Model file for the job. Use its own axes, mm. A direction names the side the tool comes from. Round coordinates to 2 decimals unless told otherwise and drop trailing zeros. Write each loop counter-clockwise with the first axis right and the second up, starting at its lowest first coordinate (ties: lowest second). Pieces come first, ordered by that corner, then holes. Notation, with made-up numbers: (-30, 55.5) - (14, 55.5) arc R21 ccw to (14, 88.5) - close; hole circle Ø8 at (71, -6.75). An arc over 180 degrees is marked (long way). Answer as a JSON object with one key per item and string values. Group by question number.
from build123d import *

# Parameters (mm, degrees)
SKETCH1_R      = 4.0005
SKETCH1_R_2    = 1.1938
EXTRUDE1_DEPTH = 1.524


with BuildPart() as part:
    # Sketch1 → Extrude1 (new body)
    with BuildSketch(Plane(origin=(0, 0, 0), x_dir=(1, 0, 0), z_dir=(0, 1, 0))):
        with BuildLine():
            Line((0, 3.175), (0, 9.525))
            Line((0, 9.525), (7.9248, 9.525))
            Line((7.9248, 9.525), (7.9248, 3.5814))
            Line((7.9248, 3.5814), (11.557, 3.5814))
            Line((11.557, 3.5814), (11.557, 9.525))
            Line((11.557, 9.525), (20.6756, 9.525))
            Line((20.6756, 9.525), (20.6756, 50.8))
            Line((20.6756, 50.8), (11.557, 50.8))
            Line((11.557, 50.8), (11.557, 56.7436))
            Line((11.557, 56.7436), (7.9248, 56.7436))
            Line((7.9248, 56.7436), (7.9248, 50.8))
            Line((7.9248, 50.8), (0, 50.8))
            Line((0, 50.8), (0, 57.15))
            ThreePointArc((0, 57.15), (0.92993597, 59.39506403), (3.175, 60.325))
            Line((3.175, 60.325), (24.638, 60.325))
            ThreePointArc((24.638, 60.325), (26.88306403, 59.39506403), (27.813, 57.15))
            Line((27.813, 57.15), (27.813, 55.9562))
            ThreePointArc((27.813, 55.9562), (28.74293597, 53.71113597), (30.988, 52.7812))
            Line((30.988, 52.7812), (49.7205, 52.7812))
            ThreePointArc((49.7205, 52.7812), (62.0268, 40.4749), (49.7205, 28.1686))
            Line((49.7205, 28.1686), (30.988, 28.1686))
            ThreePointArc((30.988, 28.1686), (28.74293597, 27.23866403), (27.813, 24.9936))
            Line((27.813, 24.9936), (27.813, 3.175))
            ThreePointArc((27.813, 3.175), (26.88306403, 0.92993597), (24.638, 0))
            Line((24.638, 0), (3.175, 0))
            ThreePointArc((3.175, 0), (0.92993597, 0.92993597), (0, 3.175))
        make_face()
        with Locations(Location((49.7205, 40.4749, 0), (0, 0, 270))):  # turned: the seam where the file's is
            Circle(SKETCH1_R, mode=Mode.SUBTRACT)
        with Locations(Location((41.3893, 40.4749, 0), (0, 0, 270))):  # turned: the seam where the file's is
            Circle(SKETCH1_R_2, mode=Mode.SUBTRACT)
        with Locations(Location((49.7205, 32.1437, 0), (0, 0, 270))):  # turned: the seam where the file's is
            Circle(SKETCH1_R_2, mode=Mode.SUBTRACT)
        with Locations(Location((58.0517, 40.4749, 0), (0, 0, 270))):  # turned: the seam where the file's is
            Circle(SKETCH1_R_2, mode=Mode.SUBTRACT)
        with Locations(Location((49.7205, 48.8061, 0), (0, 0, 270))):  # turned: the seam where the file's is
            Circle(SKETCH1_R_2, mode=Mode.SUBTRACT)
        with BuildLine():
            Line((5.842, 53.3781), (3.8608, 53.3781))
            ThreePointArc((3.8608, 53.3781), (2.2733, 54.9656), (3.8608, 56.5531))
            Line((3.8608, 56.5531), (5.842, 56.5531))
            ThreePointArc((5.842, 56.5531), (7.4295, 54.9656), (5.842, 53.3781))
        make_face(mode=Mode.SUBTRACT)
        with BuildLine():
            Line((13.6398, 6.9469), (15.621, 6.9469))
            ThreePointArc((15.621, 6.9469), (17.2085, 5.3594), (15.621, 3.7719))
            Line((15.621, 3.7719), (13.6398, 3.7719))
            ThreePointArc((13.6398, 3.7719), (12.0523, 5.3594), (13.6398, 6.9469))
        make_face(mode=Mode.SUBTRACT)
        with BuildLine():
            Line((3.8608, 3.7719), (5.842, 3.7719))
            ThreePointArc((5.842, 3.7719), (7.4295, 5.3594), (5.842, 6.9469))
            Line((5.842, 6.9469), (3.8608, 6.9469))
            ThreePointArc((3.8608, 6.9469), (2.2733, 5.3594), (3.8608, 3.7719))
        make_face(mode=Mode.SUBTRACT)
        with BuildLine():
            Line((15.621, 56.5531), (13.6398, 56.5531))
            ThreePointArc((13.6398, 56.5531), (12.0523, 54.9656), (13.6398, 53.3781))
            Line((13.6398, 53.3781), (15.621, 53.3781))
            ThreePointArc((15.621, 53.3781), (17.2085, 54.9656), (15.621, 56.5531))
        make_face(mode=Mode.SUBTRACT)
    extrude(amount=EXTRUDE1_DEPTH)


solid = part.part
(1) Pull direction X, two halves, no side cores. Call faces 1 (the cylindrical face through (0.95, 0.75, -0.91)), 2 (the flat face through (40, 1, -28.169)), 3 (the flat face through (11.557, 1, -7)), 4 (the flat face through (15, 1, -3.772)): pulls with the +X half, pulls with the -X half, needs draft (parallel to the pull), parting line crosses it, or undercut.
(2) Slice it at D-D (x = 34). Write the cut outline in (y, z), then the cut area to 3 significant figures.
(3) Slice it at B-B (x = 18.5). Write the cut outline in (y, z) (3 decimals), then the cut area to 3 significant figures.
(4) Slice it at C-C (z = -38.5). Write the cut outline in (x, y).
(5) 3-axis set-ups, long thin cutter, end or side, ignore diameter. For faces 5 (the flat face through (5, 1, -3.772)), 6 (the flat face through (16, 1, -50.8)), 7 (the flat face through (14, 1, 0)): which of +Z, -Z, +X, -X, +Y, -Y reach the whole face in a straight line?
(6) Drill centre lines: line 1 (Z direction, x = 13.5, y = 1.45) (3 decimals); line 2 (Z direction, x = 20, y = 0.9) (3 decimals); line 3 (Z direction, x = 8, y = 0.55) (3 decimals). Where is each one in solid material? Low to high. Write a range as from..to.
(7) Flat gauge pins, fed straight in: pin 1 (1.4 mm diameter, centred on x = 49.72, z = -32.14, fed in from +Y); pin 2 (0.6 mm diameter, centred on y = 1, z = -57, fed in from +X). Where does each tip first touch, or does it go through?
(8) Slice it at A-A (x = 5). Write the cut outline in (y, z) (3 decimals), then the cut area to 3 significant figures.
Answer:
{
 "1": {"face 1": "pulls with the -X half", "face 2": "needs draft", "face 3": "undercut", "face 4": "undercut"},
 "2": {"outline": "(0, -52.78) - (1.52, -52.78) - (1.52, -28.17) - (0, -28.17) - close", "area": "37.5 mm²"},
 "3": {"outline": "(0, -60.325) - (1.524, -60.325) - (1.524, -50.8) - (0, -50.8) - close; (0, -9.525) - (1.524, -9.525) - (1.524, 0) - (0, 0) - close", "area": "29.0 mm²"},
 "4": {"outline": "(20.68, 0) - (46.24, 0) - (46.24, 1.52) - (20.68, 1.52) - close; (53.2, 0) - (61.87, 0) - (61.87, 1.52) - (53.2, 1.52) - close"},
 "5": {"face 5": "+Y, -Y", "face 6": "-X, +Y, -Y", "face 7": "+Z, +X, -X, +Y, -Y"},
 "6": {"line 1": "-60.325..-56.547, -53.384..-50.8, -9.525..-6.941, -3.778..0", "line 2": "-60.325..-50.8, -9.525..0", "line 3": "-60.325..-56.744, -3.581..0"},
 "7": {"pin 1": "through", "pin 2": "x = 27.81"},
 "8": {"outline": "(0, -60.325) - (1.524, -60.325) - (1.524, -56.553) - (0, -56.553) - close; (0, -53.378) - (1.524, -53.378) - (1.524, -50.8) - (0, -50.8) - close; (0, -9.525) - (1.524, -9.525) - (1.524, -6.947) - (0, -6.947) - close; (0, -3.772) - (1.524, -3.772) - (1.524, 0) - (0, 0) - close", "area": "19.4 mm²"}
}
